Check sheet for the modelled part. Datum: model origin and axes. Units: mm. Round coordinates to 2 decimals unless told otherwise and drop trailing zeros. Loops run counter-clockwise (first coordinate to the right, second up) from the corner with the lowest first, then second, coordinate; pieces in that order, holes last. Notation, with made-up numbers: M -30.5,61.5 L 8.5,61.5 A19 cw 8.5,89.5 Z; hole C -28,-37.75 d10. An arc over 180 degrees is marked long. One line per question, with ' | ' between items. Start each with the question number.
(1) Draft check along Z on faces 1 (the face through (-21.212, -0.789, 61.537)), 2 (the face through (-33.257, -0.789, 25.66)), 3 (the face through (-33, -1, 0)). Enter one of: +Z half, -Z half, draft (parallel to the pull), parting line (faces both ways), or undercut.
(2) Section check B-B (z = 39). Record the boundary of the cut face in (x, y), and give its area (3 significant figures).
(3) Section check A-A (y = -0.65). Record the boundary of the cut face in (x, z), and give its area (3 significant figures).
(4) Section check C-C (x = -8.5). Record the boundary of the cut face in (y, z), and give its area (3 significant figures).
(5) Thickness scan on probe 1 along Z at (x, y) = (-46, -0.1); probe 2 along Z at (x, y) = (-54, -0.4); probe 3 along X at (y, z) = (-0.7, 15). Record the ranges inside material, lowest first. Write a range as [from, to].
```python
from build123d import *

# Parameters (mm, degrees)
F1_DEPTH = 1.6
F2_R     = 2.5


with BuildPart() as f1:
    # F0 (on Front) → F1 (new body)
    with BuildSketch(Plane.XZ):
        with BuildLine():
            Line((-65, 0), (0, 0))
            Line((0, 0), (-17.9164281281, 62.482010236))
            Line((-17.9164281281, 62.482010236), (-26.9059650358, 59.9043020076))
            ThreePointArc((-26.9059650358, 59.9043020076), (-33.542691422, 25.2762309724), (-65, 9.3518101738))
            Line((-65, 9.3518101738), (-65, 0))
        make_face()
    extrude(amount=F1_DEPTH)

    # F2
    f2_edges = [f1.edges().sort_by_distance(p)[0] for p in [
        (-26.905965, -0.8, 59.904302),
        (-65, -0.8, 9.35181),
    ]]
    fillet(f2_edges, radius=F2_R)


solid = f1.part
```
The answers:
1) face 1: +Z half | face 2: undercut | face 3: -Z half
2) outline: M -26.85,-1.6 L -11.18,-1.6 L -11.18,0 L -26.85,0 Z | area: 25.1 mm²
3) outline: M -65,0 L 0,0 L -17.92,62.48 L -24.6,60.57 A2.5 ccw -26.36,57.64 A40 cw -62.68,9.45 A2.5 ccw -65,6.95 Z | area: 1,740 mm²
4) outline: M -1.6,0 L 0,0 L 0,29.64 L -1.6,29.64 Z | area: 47.4 mm²
5) probe 1: [0, 14.42] | probe 2: [0, 11.03] | probe 3: [-44.99, -4.3]
